from build123d import *

# Parameters (mm, degrees)
F0_R     = 3.302
F0_R_2   = 14.3129
F1_DEPTH = 5


with BuildPart() as f1:
    # F0 (on Top) → F1 (new body)
    with BuildSketch(Plane.XY):
        with BuildLine():
            Line((-25.4, -127), (25.4, -127))
            Line((25.4, -127), (25.4, 127))
            ThreePointArc((25.4, 127), (0, 152.4), (-25.4, 127))
            Line((-25.4, 127), (-25.4, -127))
        make_face()
        Circle(F0_R, mode=Mode.SUBTRACT)
        with Locations((0, 127)):
            Circle(F0_R_2, mode=Mode.SUBTRACT)
    extrude(amount=F1_DEPTH)


solid = f1.part
Input: part model. Units: mm. Frame: model coordinates. Give positions to 0.01 mm unless a question says otherwise; leave off trailing zeros. Write each loop counter-clockwise with the first axis right and the second up, starting at its lowest first coordinate (ties: lowest second). Pieces come first, ordered by that corner, then holes. Notation, with made-up numbers: M 8.25,21.5 L 33.25,21.5 A25 ccw 33.25,44.5 Z; hole C 16.5,41.25 d4. An arc over 180 degrees is marked long. Use one line per item in the form item = value.
1. Mould query, pull axis Y, two halves, no side actions, for faces 1 (the face through (25.4, -2, 2)), 2 (the face through (3.05, -1.26, 2.46)), 3 (the face through (0.559, 152.394, 2.465)), 4 (the face through (-1.86, 141.19, 2.46)). Classes: released by +Y, released by -Y, zero draft, split by the parting line, or undercut.
Outcome:
face_1 = zero draft
face_2 = undercut
face_3 = released by +Y
face_4 = undercut
2. Cut plane B-B on x = 0. Return loops of the section in (y, z), and give its area (3 significant figures).
Outcome:
outline = M -127,0 L -3.3,0 L -3.3,5 L -127,5 Z; M 3.3,0 L 112.69,0 L 112.69,5 L 3.3,5 Z; M 141.31,0 L 152.4,0 L 152.4,5 L 141.31,5 Z
area = 1,220 mm²
3. Cut plane A-A on y = 0. Return loops of the section in (x, z).
Outcome:
outline = M -25.4,0 L -3.3,0 L -3.3,5 L -25.4,5 Z; M 3.3,0 L 25.4,0 L 25.4,5 L 3.3,5 Z
4. Ray query, L1, parallel to Y at x = 0, z = 3.7; L2, parallel to X at y = 126, z = 1.5; L3, parallel to Y at x = -2, z = 3.6. Return the intervals inside material, ascending.
Outcome:
L1 = -127 to -3.3, 3.3 to 112.69, 141.31 to 152.4
L2 = -25.4 to -14.28, 14.28 to 25.4
L3 = -127 to -2.63, 2.63 to 112.83, 141.17 to 152.32
5. Cut plane D-D on x = -12. Return loops of the section in (y, z), and give its area (3 significant figures).
Outcome:
outline = M -127,0 L 119.2,0 L 119.2,5 L -127,5 Z; M 134.8,0 L 149.39,0 L 149.39,5 L 134.8,5 Z
area = 1,300 mm²
6. Cut plane C-C on z = 2.9. Return loops of the section in (x, y), and give its area (3 significant figures).
Outcome:
outline = M -25.4,-127 L 25.4,-127 L 25.4,127 A25.4 ccw -25.4,127 Z; hole C 0,127 d28.63; hole C 0,0 d6.6
area = 13,200 mm²
